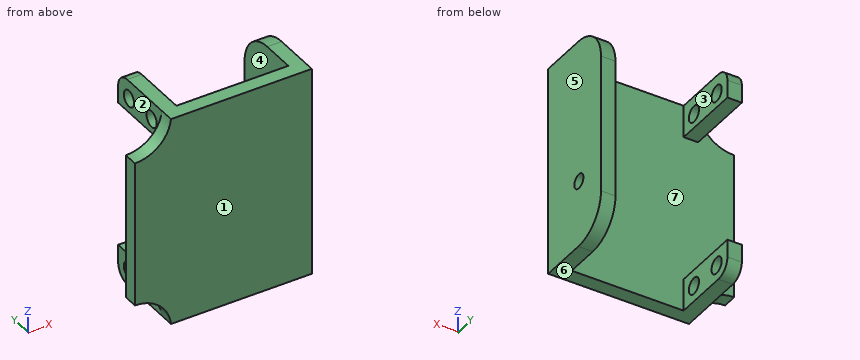
from build123d import *

# Parameters (mm, degrees)
BOSS_EXTRUDE1_DEPTH = 4
SKETCH2_W           = 8.95
SKETCH2_H           = 19.3
SKETCH2_R           = 2.25
BOSS_EXTRUDE2_DEPTH = 4
FILLET1_R           = 10
FILLET2_R           = 4
SKETCH3_W           = 58.4
SKETCH3_H           = 19.3
SKETCH3_R           = 2
BOSS_EXTRUDE3_DEPTH = 4
FILLET3_R           = 10


with BuildPart() as part:
    # Sketch1 → Boss-Extrude1 (new body)
    with BuildSketch(Plane(origin=(0, 0, 0), x_dir=(1, 0, 0), z_dir=(0, 1, 0))):
        Polygon((-49, 49.45), (-39, 49.45), (-39, 58.4), (0, 58.4), (0, 0), (-39, 0), (-39, 8.95), (-49, 8.95), align=None)
    extrude(amount=BOSS_EXTRUDE1_DEPTH)

    # Sketch2 → Boss-Extrude2 (add)
    # profile 1 of 2: a face of its own
    with BuildSketch(Plane.ZY.offset(39)):
        with Locations((-4.475, 13.65)):
            Rectangle(SKETCH2_W, SKETCH2_H)
        with Locations((-5, 18.55)):
            Circle(SKETCH2_R, mode=Mode.SUBTRACT)
        with Locations((-5, 8.55)):
            Circle(SKETCH2_R, mode=Mode.SUBTRACT)
    # profile 2 of 2: a face of its own
    with BuildSketch(Plane.ZY.offset(39)):
        with Locations((-53.925, 13.65)):
            Rectangle(SKETCH2_W, SKETCH2_H)
        with Locations((-54, 18.55)):
            Circle(SKETCH2_R, mode=Mode.SUBTRACT)
        with Locations((-54, 8.55)):
            Circle(SKETCH2_R, mode=Mode.SUBTRACT)
    extrude(amount=-BOSS_EXTRUDE2_DEPTH)

    # Fillet1
    # the kernel refuses this fillet: 10 mm, written as the material it adds along each edge
    with BuildSketch(Plane(origin=(-39, 0, -49.45), x_dir=(-1, 0, 0), z_dir=(0, 1, 0))) as fillet1_piece_1:
        with BuildLine():
            CenterArc((9.944722218, -10), FILLET1_R, 90, 83.97283344)
            Line((0, -8.95), (0, 0))
            Line((0, 0), (9.944722218, 0))
        make_face()
    extrude(amount=4)
    with BuildSketch(Plane(origin=(-39, 0, -8.95), x_dir=(0, 0, 1), z_dir=(0, 1, 0))) as fillet1_piece_2:
        with BuildLine():
            CenterArc((10, -9.944722218), FILLET1_R, 96.02716656, 83.97283344)
            Line((0, -9.944722218), (0, 0))
            Line((0, 0), (8.95, 0))
        make_face()
    extrude(amount=4)

    # Fillet2
    fillet2_edges = [part.edges().sort_by_distance(p)[0] for p in [
        (-37, 23.3, 0),
        (-37, 23.3, -58.4),
    ]]
    fillet(fillet2_edges, radius=FILLET2_R)

    # Sketch3 → Boss-Extrude3 (add)
    with BuildSketch(Plane(origin=(0, 0, 0), x_dir=(0, 0, -1), z_dir=(1, 0, 0))):
        with Locations((29.2, 13.65)):
            Rectangle(SKETCH3_W, SKETCH3_H)
        with Locations((39.95, 13.55)):
            Circle(SKETCH3_R, mode=Mode.SUBTRACT)
    extrude(amount=-BOSS_EXTRUDE3_DEPTH)

    # Fillet3
    fillet3_edges = [part.edges().sort_by_distance(p)[0] for p in [
        (-2, 23.3, 0),
        (-2, 23.3, -58.4),
    ]]
    fillet(fillet3_edges, radius=FILLET3_R)


solid = part.part
Part model, mm, in its own coordinate system. Face numbers are marked on the shaded views. A direction names the side the tool comes from. Give positions to 0.01 mm unless a question says otherwise; leave off trailing zeros. Loops run counter-clockwise (first coordinate to the right, second up) from the corner with the lowest first, then second, coordinate; pieces in that order, holes last.
(1) Band-saw the part on D-D (y = 18.55). Write the cut outline in (x, z), and give its area (3 significant figures).
Return value:
outline: (-39, -58.4) - (-35, -58.4) - (-35, -56.25) - (-39, -56.25) - close; (-39, -51.75) - (-35, -51.75) - (-35, -49.45) - (-39, -49.45) - close; (-39, -8.95) - (-35, -8.95) - (-35, -7.25) - (-39, -7.25) - close; (-39, -2.75) - (-35, -2.75) - (-35, 0) - (-39, 0) - close; (-4, -56.91) - (0, -56.91) - (0, -1.49) - (-4, -1.49) - close
area: 257 mm2
(2) Pull direction X, two halves, no side cores. Call the marked faces 4, 5, 6 and 7: pulls with the +X half, pulls with the -X half, needs draft (parallel to the pull), parting line crosses it, or undercut.
Return value:
face 4: undercut
face 5: pulls with the +X half
face 6: needs draft
face 7: undercut
(3) Band-saw the part on A-A (y = 8.55). Write the cut outline in (x, z), and give its area (3 significant figures).
Return value:
outline: (-39, -58.4) - (-35, -58.4) - (-35, -56.25) - (-39, -56.25) - close; (-39, -51.75) - (-35, -51.75) - (-35, -49.45) - (-39, -49.45) - close; (-39, -8.95) - (-35, -8.95) - (-35, -7.25) - (-39, -7.25) - close; (-39, -2.75) - (-35, -2.75) - (-35, 0) - (-39, 0) - close; (-4, -58.4) - (0, -58.4) - (0, 0) - (-4, 0) - close
area: 269 mm2
(4) Pin check, flat tips, straight feed: pin 1 (6 mm diameter, centred on y = 8.55, z = -5, fed in from -X); pin 2 (4 mm diameter, centred on y = 8.55, z = -54, fed in from -X); pin 3 (22.5 mm diameter, centred on x = -29.5, z = -24.5, fed in from +Y). Stop position of each tip, or through.
Return value:
pin 1: stops at x = -39
pin 2: stops at x = -4
pin 3: stops at y = 4
(5) Band-saw the part on C-C (z = -27). Write the cut outline in (x, y).
Return value:
outline: (-49, 0) - (0, 0) - (0, 23.3) - (-4, 23.3) - (-4, 4) - (-49, 4) - close
(6) Drill centre lines: line 1 along Y through (x, z) = (-36.35, -54); line 2 along X through (y, z) = (18.5, -50.5); line 3 along X through (y, z) = (20, -40.5). Where is each one in solid material? Low to high.
Return value:
line 1: y = 0 to 6.3, 10.8 to 16.3, 20.8 to 23.3
line 2: x = -39 to -35, -4 to 0
line 3: x = -4 to 0
(7) Band-saw the part on B-B (z = -39.95). Write the cut outline in (x, y), and give its area (3 significant figures).
Return value:
outline: (-49, 0) - (0, 0) - (0, 11.55) - (-4, 11.55) - (-4, 4) - (-49, 4) - close; (-4, 15.55) - (0, 15.55) - (0, 23.3) - (-4, 23.3) - close
area: 257 mm2
(8) 3-axis set-ups, long thin cutter, end or side, ignore diameter. For the marked faces 1, 2 and 3: which of +Z, -Z, +X, -X, +Y, -Y reach the whole face in a straight line?
Return value:
face 1: +Z, -Z, +X, -X, -Y
face 2: +Z, -Z, -X, +Y
face 3: +Z, -Z, +Y
